Verification items for the finished model (mm, model axes). A direction names the side the tool comes from. Give positions to 0.01 mm unless a question says otherwise; leave off trailing zeros. Write each loop counter-clockwise with the first axis right and the second up, starting at its lowest first coordinate (ties: lowest second). Pieces come first, ordered by that corner, then holes. Notation, with made-up numbers: (-6.75, -9.75) -> (38.25, -9.75) arc R35 ccw to (38.25, 27.25) -> close; hole circle Ø4 at (73.25, 74). An arc over 180 degrees is marked (long way). Use CSV: the item, a comma, the result in double quotes. Start each with the question number.
```python
from build123d import *

# Parameters (mm, degrees)
SKETCH2_R                = 12.5
BOSS_EXTRUDE1_DEPTH      = 10
BOSS_EXTRUDE3_DEPTH      = 5
BOSS_EXTRUDE3_DEPTH_BACK = 15
SKETCH4_R                = 1
CUT_EXTRUDE1_DEPTH       = 20
SKETCH5_R                = 3
CUT_EXTRUDE2_DEPTH       = 5
CUT_EXTRUDE3_START       = -10
SKETCH6_R                = 3
CUT_EXTRUDE3_DEPTH       = 10


with BuildPart() as part:
    # Sketch2 → Boss-Extrude1 (new body)
    with BuildSketch(Plane(origin=(0, 0, 0), x_dir=(0, 0, -1), z_dir=(1, 0, 0))):
        Circle(SKETCH2_R)
    extrude(amount=BOSS_EXTRUDE1_DEPTH)

    # Sketch3 → Boss-Extrude3 (add, two sides: drawn at the far end of the back side and taken through both)
    with BuildSketch(Plane.ZY.offset(-BOSS_EXTRUDE3_DEPTH_BACK)):
        Polygon((10.823922003, 0), (7.653668647, 7.653668647), (0, 10.823922003), (-7.653668647, 7.653668647), (-10.823922003, 0), (-7.653668647, -7.653668647), (0, -10.823922003), (7.653668647, -7.653668647), align=None)
    extrude(amount=BOSS_EXTRUDE3_DEPTH + BOSS_EXTRUDE3_DEPTH_BACK)

    # Sketch4 → Cut-Extrude1 (cut)
    with BuildSketch(Plane.ZY.offset(5)):
        with Locations((1.913417162, 4.619397663)):
            Circle(SKETCH4_R)
        with Locations((-1.913417162, -4.619397663)):
            Circle(SKETCH4_R)
    extrude(amount=-CUT_EXTRUDE1_DEPTH, mode=Mode.SUBTRACT)

    # Sketch5 → Cut-Extrude2 (cut)
    with BuildSketch(Plane.ZY.offset(5)):
        with Locations((-1.913417162, -4.619397663)):
            Circle(SKETCH5_R)
        with Locations((1.913417162, 4.619397663)):
            Circle(SKETCH5_R)
    extrude(amount=-CUT_EXTRUDE2_DEPTH, mode=Mode.SUBTRACT)

    # Sketch6 → Cut-Extrude3 (cut)
    with BuildSketch(Plane(origin=(15, 0, 0), x_dir=(0, 0, -1), z_dir=(1, 0, 0)).offset(CUT_EXTRUDE3_START)):
        with Locations(Location((1.913417162, -4.619397663, 0), (0, 0, 180))):
            Circle(SKETCH6_R)
        with Locations(Location((-1.913417162, 4.619397663, 0), (0, 0, 180))):
            Circle(SKETCH6_R)
    extrude(amount=CUT_EXTRUDE3_DEPTH, mode=Mode.SUBTRACT)


solid = part.part
```
(1) Section check A-A on x = 13.5. Record the cut outline in (y, z).
(2) Thickness scan on line 1 (X direction, y = 4, z = -9.25); line 2 (Y direction, x = 11.75, z = -2); line 3 (Z direction, x = 13.75, y = -2.5). Record the ranges inside material, lowest first. Write a range as from..to.
(3) Section check B-B on z = 4. Record the cut outline in (x, y).
(4) Set-up check for faces 4 (the face through (12.535, 3.88, -9.217)), 5 (the face through (-2.465, -3.773, -9.261)), 6 (the face through (5, 5, 3)), 7 (the face through (0, 10.244, -1.794)): record each of +Z, -Z, +X, -X, +Y, -Y from which the full face is reachable in a straight line by a thin tool's end or side.
(5) Draft check along Z on faces 1 (the face through (2.465, -3.628, -2.044)), 2 (the face through (10, 10.244, -1.794)), 3 (the face through (-2.465, 9.261, -3.773)). Enter one of: released by +Z, released by -Z, zero draft, split by the parting line, or undercut.
(6) Section check D-D on z = 10. Record the cut outline in (x, y).
(7) Go/stop test with flat-tipped pins: pin 1 (2.5 mm diameter, centred on y = 4.62, z = 1.91, fed in from +X); pin 2 (5 mm diameter, centred on x = 6.5, z = -1.5, fed in from +Y); pin 3 (3 mm diameter, centred on y = 4, z = 2.5, fed in from -X); pin 4 (4 mm diameter, centred on x = 3.5, y = 7.5, fed in from +Z) (3 decimals). Record where each tip stops, or that it passes through.
(8) Section check C-C on y = -0.5. Record the cut outline in (x, z).
Data:
1,outline,"(-10.82, 0) -> (-7.65, -7.65) -> (0, -10.82) -> (7.65, -7.65) -> (10.82, 0) -> (7.65, 7.65) -> (0, 10.82) -> (-7.65, 7.65) -> close; hole circle Ø6 at (-4.62, -1.91); hole circle Ø6 at (4.62, 1.91)"
2,line 1,"x = 0..10"
2,line 2,"y = -10..-7.62, -1.62..10"
2,line 3,"z = -9.79..-4.04, 0.21..9.79"
3,outline,"(-5, -9.17) -> (0, -9.17) -> (0, -11.84) -> (10, -11.84) -> (10, -9.17) -> (15, -9.17) -> (15, 2.46) -> (5, 2.46) -> (5, 6.77) -> (15, 6.77) -> (15, 9.17) -> (10, 9.17) -> (10, 11.84) -> (0, 11.84) -> (0, 9.17) -> (-5, 9.17) -> (-5, 6.77) -> (0, 6.77) -> (0, 2.46) -> (-5, 2.46) -> close"
4,face 4,"-Z, +X, +Y"
4,face 5,"-Z, -X, -Y"
4,face 6,"+X"
4,face 7,"-X"
5,face 1,"undercut"
5,face 2,"zero draft"
5,face 3,"released by -Z"
6,outline,"(-5, -1.99) -> (0, -1.99) -> (0, -7.5) -> (10, -7.5) -> (10, -1.99) -> (15, -1.99) -> (15, 1.99) -> (10, 1.99) -> (10, 7.5) -> (0, 7.5) -> (0, 1.99) -> (-5, 1.99) -> close"
7,pin 1,"stops at x = 5"
7,pin 2,"stops at y = 12.5"
7,pin 3,"stops at x = 0"
7,pin 4,"stops at z = 11.225"
8,outline,"(-5, -10.62) -> (0, -10.62) -> (0, -12.49) -> (10, -12.49) -> (10, -10.62) -> (15, -10.62) -> (15, 10.62) -> (10, 10.62) -> (10, 12.49) -> (0, 12.49) -> (0, 10.62) -> (-5, 10.62) -> close"
